from build123d import *

# Parameters (mm, degrees)
SKETCH1_R        = 20.55
BASE_DEPTH       = 27.4955
TOP_DEPTH        = 38.7223
SKETCH3_R        = 2
MOUNTING_DEPTH   = 6.35
NPTF_DEPTH       = 76.952904361
NPTF_DEPTH_BACK  = 76.952904361
SKETCH4_R        = 5.55625
SKETCH5_R        = 12.7
SKETCH5_R_2      = 11.1125
CABLE_TUBE_DEPTH = 18.0086


with BuildPart() as part:
    # Sketch1 → BASE (new body)
    with BuildSketch(Plane(origin=(0, 0, 0), x_dir=(1, 0, 0), z_dir=(0, 1, 0))):
        with Locations(Location((0, 0, 0), (0, 0, 270))):
            Circle(SKETCH1_R)
    extrude(amount=BASE_DEPTH)

    # Sketch2 → TOP (add)
    with BuildSketch(Plane(origin=(0, 27.4955, 0), x_dir=(1, 0, 0), z_dir=(0, 1, 0))):
        with BuildLine():
            Line((-20.55, 0), (-20.55, -31.012))
            Line((-20.55, -31.012), (20.55, -31.012))
            Line((20.55, -31.012), (20.55, 0))
            ThreePointArc((20.55, 0), (0, 20.55), (-20.55, 0))
        make_face()
    extrude(amount=TOP_DEPTH)

    # Sketch3 → MOUNTING (cut)
    with BuildSketch(Plane.XZ):
        with Locations(Location((11.2, 11.2, 0), (0, 0, 270))):
            Circle(SKETCH3_R)
        with Locations(Location((-11.2, -11.2, 0), (0, 0, 270))):
            Circle(SKETCH3_R)
    extrude(amount=-MOUNTING_DEPTH, mode=Mode.SUBTRACT)

    # Sketch4 → NPTF (cut, two sides: drawn at the far end of the back side and taken through both)
    with BuildSketch(Plane(origin=(0, 0, 0), x_dir=(0, 0, -1), z_dir=(1, 0, 0)).offset(-NPTF_DEPTH_BACK)):
        with Locations((0, 8.6)):
            Circle(SKETCH4_R)
    extrude(amount=NPTF_DEPTH + NPTF_DEPTH_BACK, mode=Mode.SUBTRACT)

    # Sketch5 → CABLE_TUBE (add)
    with BuildSketch(Plane.XY.offset(31.012)):
        with Locations(Location((0, 46.85665, 0), (0, 0, 180))):
            Circle(SKETCH5_R)
        with Locations((0, 46.85665)):
            Circle(SKETCH5_R_2, mode=Mode.SUBTRACT)
    extrude(amount=CABLE_TUBE_DEPTH)


solid = part.part
Geometry check sheet. Reference: the model listing, model coordinates, mm. A direction names the side the tool comes from. Give positions to 0.01 mm unless a question says otherwise; leave off trailing zeros. Write each loop counter-clockwise with the first axis right and the second up, starting at its lowest first coordinate (ties: lowest second). Pieces come first, ordered by that corner, then holes. Notation, with made-up numbers: M -27.5,47.25 L 18.5,47.25 A9 ccw 18.5,60.25 Z; hole C 35,-31 d1. An arc over 180 degrees is marked long. One line per question, with ' | ' between items.
1. Cross-section at C-C (z = -11.2). Enter the section's corners in (x, y), plus the area to 3 significant figures.
Ans:
outline: M -17.23,0 L -13.2,0 L -13.2,6.35 L -9.2,6.35 L -9.2,0 L 17.23,0 L 17.23,66.22 L -17.23,66.22 Z | area: 2,260 mm2
2. Cross-section at D-D (y = 49.5). Enter the section's corners in (x, z), plus the area to 3 significant figures.
Ans:
outline: M -20.55,0 A20.55 ccw 20.55,0 L 20.55,31.01 L 12.42,31.01 L 12.42,49.02 L 10.79,49.02 L 10.79,31.01 L -10.79,31.01 L -10.79,49.02 L -12.42,49.02 L -12.42,31.01 L -20.55,31.01 Z | area: 2,000 mm2
3. Scan lines: line 1 along Y through (x, z) = (11, 0); line 2 along X through (y, z) = (24.5, -0.5); line 3 along Y through (x, z) = (-7, 42.5). Record each from-to range of solid material in increasing order. Write a range as from..to.
Ans:
line 1: 0..3.04, 14.16..66.22 | line 2: -20.54..20.54 | line 3: 36.26..38.23, 55.49..57.45
4. Cross-section at B-B (y = 8.6). Enter the section's corners in (x, z), plus the area to 3 significant figures.
Ans:
outline: M -19.78,-5.56 A20.55 ccw 19.78,-5.56 Z; M -19.78,5.56 L 19.78,5.56 A20.55 ccw Z | area: 876 mm2
5. Gauge pin test, flat ends, axial feed: pin 1 (12 mm diameter, centred on x = 3, y = 48.5, fed in from -Z); pin 2 (6.5 mm diameter, centred on x = -3.5, y = 41.5, fed in from +Z); pin 3 (1.2 mm diameter, centred on x = 11, z = 10.5, fed in from -Y); pin 4 (10 mm diameter, centred on y = 8.6, z = 0, fed in from -X). Record the tip position at first contact, or that the pin passes through.
Ans:
pin 1: z = -20.55 | pin 2: z = 31.01 | pin 3: y = 6.35 | pin 4: through
6. Set-up check for faces 4 (the face through (10.434, 3.131, 9.353)), 5 (the face through (20.55, 47, 16)), 6 (the face through (-5.86, 58.124, 39.89)), 7 (the face through (0, 66.218, 5)), 8 (the face through (0, 27.496, 22)): record each of +Z, -Z, +X, -X, +Y, -Y from which the full face is reachable in a straight line by a thin tool's end or side.
Ans:
face 4: -Y | face 5: +Z, -Z, +X, +Y, -Y | face 6: +Z | face 7: +Z, -Z, +X, -X, +Y | face 8: +Z, -Y
7. Cross-section at A-A (x = -4). Enter the section's corners in (y, z), plus the area to 3 significant figures.
Ans:
outline: M 0,-20.16 L 66.22,-20.16 L 66.22,31.01 L 58.91,31.01 L 58.91,49.02 L 57.22,49.02 L 57.22,31.01 L 36.49,31.01 L 36.49,49.02 L 34.8,49.02 L 34.8,31.01 L 27.5,31.01 L 27.5,20.16 L 0,20.16 Z; hole C 8.6,0 d11.11 | area: 3,050 mm2
8. Mould release check, pull along Y, two halves, no side actions. Record for faces 1 (the face through (-11, 6.35, -11)), 2 (the face through (-0.9, 58.1, 49.021)), 3 (the face through (-0.29, 10.27, -5.3)): released by +Y, released by -Y, zero draft, split by the parting line, or undercut.
Ans:
face 1: released by -Y | face 2: zero draft | face 3: undercut
